from build123d import *

# Parameters (mm, degrees)
EXTRUDE_1_DEPTH = 18
SKETCH_2_R      = 18
EXTRUDE_2_DEPTH = 15
EXTRUDE_3_DEPTH = 9


with BuildPart() as part:
    # Эскиз1 → Бобышка-Вытянуть1 (new body)
    with BuildSketch(Plane.XY):
        with BuildLine():
            Line((513.746536265, 159.110381716), (518.975806012, 171.093022728))
            ThreePointArc((518.975806012, 171.093022728), (534.766582533, 179.569802198), (541.069644925, 196.347043265))
            Line((541.069644925, 196.347043265), (535.885484235, 223.616162023))
            ThreePointArc((535.885484235, 223.616162023), (570.695429585, 265.667333265), (605.505374934, 223.616162023))
            Line((605.505374934, 223.616162023), (600.321214244, 196.347043265))
            ThreePointArc((600.321214244, 196.347043265), (606.624276637, 179.569802198), (622.415053158, 171.093022728))
            Line((622.415053158, 171.093022728), (627.644322904, 159.110381716))
            ThreePointArc((627.644322904, 159.110381716), (570.695429585, 128.269815911), (513.746536265, 159.110381716))
        make_face()
    extrude(amount=EXTRUDE_1_DEPTH)


with BuildPart() as body_2:
    # Эскиз2 → Бобышка-Вытянуть2 (new body)
    with BuildSketch(Plane.XY.offset(18)):
        with Locations((570.695429585, 237.392875312)):
            Circle(SKETCH_2_R)
    extrude(amount=EXTRUDE_2_DEPTH)


with BuildPart() as body_3:
    # Эскиз4 → Бобышка-Вытянуть3 (new body)
    with BuildSketch(Plane.XY.offset(33)):
        with BuildLine():
            Line((539.695429585, 155.14675651), (539.695429585, 237.392875312))
            ThreePointArc((539.695429585, 237.392875312), (570.695429585, 268.392875312), (601.695429585, 237.392875312))
            Line((601.695429585, 237.392875312), (601.695429585, 155.14675651))
            ThreePointArc((601.695429585, 155.14675651), (570.695429585, 124.14675651), (539.695429585, 155.14675651))
        make_face()
    extrude(amount=EXTRUDE_3_DEPTH)

    # Combine 3: union part, body 2
    add(part.part)
    add(body_2.part)


solid = body_3.part
Geometry check sheet. Reference: the model listing, model coordinates, mm. A direction names the side the tool comes from. Round coordinates to 2 decimals unless told otherwise and drop trailing zeros. Order: outer loops, then holes, each group sorted by start corner. A loop starts at its lowest first (then second) coordinate and runs counter-clockwise, first axis right, second up. Notation, with made-up numbers: M 42,62.5 L 72,62.5 A21 ccw 72,71.5 Z; hole C -1,45 d3. An arc over 180 degrees is marked long. Write each question's results on one line, items separated by ' | '. Start each with the question number.
1. Cross-section at C-C on y = 200.5. Record the boundary of the cut face in (x, z), plus the area to 3 significant figures.
2. Set-up check for faces 4 (the face through (538.514, 209.791, 8.874)), 5 (the face through (606.46, 179.76, 8.87)), 6 (the face through (566.79, 219.82, 25.4)), 7 (the face through (571.64, 128.276, 8.874)), 8 (the face through (571.377, 124.154, 37.437)): record each of +Z, -Z, +X, -X, +Y, -Y from which the full face is reachable in a straight line by a thin tool's end or side.
3. Go/stop test with flat-tipped pins: P1, Ø1.5, axis at x = 563.5, z = 9.5, coming from the -Y side; P2, Ø10, axis at x = 612.5, z = 18, coming from the -Y side; P3, Ø6, axis at y = 188, z = 34.5, coming from the -X side. Record where each tip stops, or that it passes through.
4. Cross-section at D-D on y = 234.5. Record the boundary of the cut face in (x, z), plus the area to 3 significant figures.
5. Draft check along Z on faces 1 (the face through (601.695, 197, 37)), 2 (the face through (571, 197, 42)), 3 (the face through (571, 181, 33)). Enter one of: pulls with the +Z half, pulls with the -Z half, needs draft (parallel to the pull), parting line crosses it, or undercut.
6. Cross-section at B-B on z = 7. Record the boundary of the cut face in (x, y), plus the area to 3 significant figures.
7. Cross-section at A-A on x = 543.5. Record the boundary of the cut face in (y, z), plus the area to 3 significant figures.
8. Material ranges on L1, parallel to Z at x = 553.5, y = 253; L2, parallel to X at y = 162, z = 38.5; L3, parallel to Z at x = 535, y = 142, recorded low to high. Write a range as from..to.
Resolved:
1) outline: M 539.7,33 L 601.7,33 L 601.7,42 L 539.7,42 Z; M 540.28,0 L 601.11,0 L 601.11,18 L 540.28,18 Z | area: 1,650 mm2
2) face 4: -Z, -X | face 5: -Z, +X | face 6: none | face 7: -Z, -Y | face 8: +Z, -Y
3) P1: y = 128.58 | P2: y = 139.09 | P3: x = 539.7
4) outline: M 535.52,0 L 605.87,0 L 605.87,18 L 588.46,18 L 588.46,33 L 601.7,33 L 601.7,42 L 539.7,42 L 539.7,33 L 552.93,33 L 552.93,18 L 535.52,18 Z | area: 2,360 mm2
5) face 1: needs draft | face 2: pulls with the +Z half | face 3: undercut
6) outline: M 513.75,159.11 A68 ccw 627.64,159.11 L 622.42,171.09 A25.48 cw 600.32,196.35 L 605.51,223.62 A35.43 ccw long 535.89,223.62 L 541.07,196.35 A25.48 cw 518.98,171.09 Z | area: 9,740 mm2
7) outline: M 133.94,0 L 252.95,0 L 252.95,18 L 133.94,18 Z; M 140.27,33 L 252.27,33 L 252.27,42 L 140.27,42 Z | area: 3,150 mm2
8) L1: 0..18, 33..42 | L2: 539.7..601.7 | L3: 0..18
